from build123d import *

# Parameters (mm, degrees)
SKETCH1_W           = 8
SKETCH1_H           = 10
BOSS_EXTRUDE1_DEPTH = 122
SKETCH2_W           = 3.8
SKETCH2_H           = 3.8
BOSS_EXTRUDE2_DEPTH = 1.8
SKETCH3_W           = 3.8
SKETCH3_H           = 3.8
BOSS_EXTRUDE3_DEPTH = 1.8


with BuildPart() as part:
    # Sketch1 → Boss-Extrude1 (new body)
    with BuildSketch(Plane.XY):
        with Locations((4, 5)):
            Rectangle(SKETCH1_W, SKETCH1_H)
    extrude(amount=BOSS_EXTRUDE1_DEPTH)

    # Sketch2 → Boss-Extrude2 (add)
    with BuildSketch(Plane(origin=(0, 0, 0), x_dir=(-1, 0, 0), z_dir=(0, 0, -1))):
        with Locations((-4, 4)):
            Rectangle(SKETCH2_W, SKETCH2_H)
    extrude(amount=BOSS_EXTRUDE2_DEPTH)

    # Sketch3 → Boss-Extrude3 (add)
    with BuildSketch(Plane.XY.offset(122)):
        with Locations((4, 4)):
            Rectangle(SKETCH3_W, SKETCH3_H)
    extrude(amount=BOSS_EXTRUDE3_DEPTH)


solid = part.part
Read the model definition and answer for the solid it produces. Units are mm, in the model's axes. Round coordinates to 2 decimals unless told otherwise and drop trailing zeros. Order: outer loops, then holes, each group sorted by start corner. A loop starts at its lowest first (then second) coordinate and runs counter-clockwise, first axis right, second up.
1) A straight line is drawn through the part: L1, parallel to Z at x = 6.75, y = 6.25. Find the intervals that lie inside material, in ascending order.
2) The part is cut by section B-B on x = 4.75. Write down the section's boundary in (y, z), plus the area to 3 significant figures.
3) Flat-ended cylindrical pins translate along their axes: pin 1 (3 mm diameter, centred on x = 5, z = 70, fed in from -Y); pin 2 (0.9 mm diameter, centred on x = 3.5, z = -1, fed in from -Y); pin 3 (1.4 mm diameter, centred on x = 3.5, z = -1, fed in from +Y); pin 4 (4 mm diameter, centred on x = 4.5, y = 9, fed in from -Z). Find the tip coordinate at first contact, or state that the pin passes through.
4) The mould has two halves that part along Z. Classify faces 1 (the face through (4, 4, -1.8)), 2 (the face through (4, 4, 123.8)), 3 (the face through (4, 0, 60)): released by +Z, released by -Z, zero draft, split by the parting line, or undercut.
5) The part is cut by section A-A on y = 4.75. Write down the section's boundary in (x, z), plus the area to 3 significant figures.
Resolved:
1. L1: z = 0 to 122
2. outline: (0, 0) - (2.1, 0) - (2.1, -1.8) - (5.9, -1.8) - (5.9, 0) - (10, 0) - (10, 122) - (5.9, 122) - (5.9, 123.8) - (2.1, 123.8) - (2.1, 122) - (0, 122) - close
2. area: 1,230 mm2
3. pin 1: stops at y = 0
3. pin 2: stops at y = 2.1
3. pin 3: stops at y = 5.9
3. pin 4: stops at z = 0
4. face 1: released by -Z
4. face 2: released by +Z
4. face 3: zero draft
5. outline: (0, 0) - (2.1, 0) - (2.1, -1.8) - (5.9, -1.8) - (5.9, 0) - (8, 0) - (8, 122) - (5.9, 122) - (5.9, 123.8) - (2.1, 123.8) - (2.1, 122) - (0, 122) - close
5. area: 990 mm2
